Here's how the part is built. I have some questions about the finished solid (model axes, mm). Face numbers are marked on the shaded views. A direction names the side the tool comes from. Coordinates: 2 decimals unless noted, no trailing zeros. Order: outer loops, then holes, each group sorted by start corner. A loop starts at its lowest first (then second) coordinate and runs counter-clockwise, first axis right, second up. Notation, with made-up numbers: (14.25, 45.5) - (52.25, 45.5) arc R6 ccw to (52.25, 53.5) - close; hole circle Ø9 at (-11.5, 13). An arc over 180 degrees is marked (long way). Answer as CSV lines item,"result". Start each with the question number.
Item 1: I'm going to push flat-ended pins straight in: pin 1 (10 mm diameter, centred on y = -380.5, z = 182.5, fed in from -X); pin 2 (12 mm diameter, centred on x = 169.5, y = -310, fed in from -Z); pin 3 (8 mm diameter, centred on x = 40, y = -347, fed in from +Z). Where does each tip first touch, or does it pass through?
Item 2: I need wall thicknesses on line 1 (Z direction, x = 0, y = -113); line 2 (X direction, y = -492.5, z = 32); line 3 (Z direction, x = 149.5, y = -647.7). Which ranges of each line are inside material? Lowest first, please.
Item 3: Imagine slicing it at C-C on x = 0. List the corners of the cut face in (y, z) for me.
Item 4: On a 3-axis mill with a long thin cutter (end or side, diameter ignored), from which of +Z, -Z, +X, -X, +Y, -Y can I reach the whole of each face in a straight line? I mean the marked faces 1, 2 and 3. Say none if no direction works.
Item 5: Imagine slicing it at D-D on z = 0. List the corners of the cut face in (x, y) for me, and give its area (3 significant figures).
Item 6: We'd pull the mould along Z, two halves only. Please class the marked faces 4, 5, 6 and 7: pulls with the +Z half, pulls with the -Z half, needs draft (parallel to the pull), parting line crosses it, or undercut.
Item 7: Imagine slicing it at A-A on y = -647.7. List the corners of the cut face in (x, z) for me.
Item 8: Imagine slicing it at B-B on y = -482. List the corners of the cut face in (x, z) for me.
from build123d import *

# Parameters (mm, degrees)
F0_R     = 254
F0_R_2   = 127
F1_DEPTH = 254
F2_R     = 254
F3_DEPTH = 127
F4_W     = 112.5292529635
F4_H     = 228.6
F5_DEPTH = 381
F6_R     = 38.1
F7_DEPTH = 480.8302529635


with BuildPart() as f1:
    # F0 (on Front) → F1 (new body)
    with BuildSketch(Plane.XZ):
        Circle(F0_R)
        Circle(F0_R_2, mode=Mode.SUBTRACT)
    extrude(amount=F1_DEPTH)

    # F2 (on face) → F3 (join)
    with BuildSketch(Plane.XZ.offset(254)):
        Circle(F2_R)
    extrude(amount=F3_DEPTH)

    # F4 (on face) → F5 (join)
    with BuildSketch(Plane.XZ.offset(381)):
        with Locations((-170.5646264818, 0)):
            Rectangle(F4_W, F4_H)
        with Locations((170.5646264818, 0)):
            Rectangle(F4_W, F4_H)
    extrude(amount=F5_DEPTH)

    # F6 (on face) → F7 (cut, through all)
    with BuildSketch(Plane.YZ.offset(226.8292529635)):
        with Locations((-647.7, 0)):
            Circle(F6_R)
    extrude(amount=-F7_DEPTH, mode=Mode.SUBTRACT)


solid = f1.part
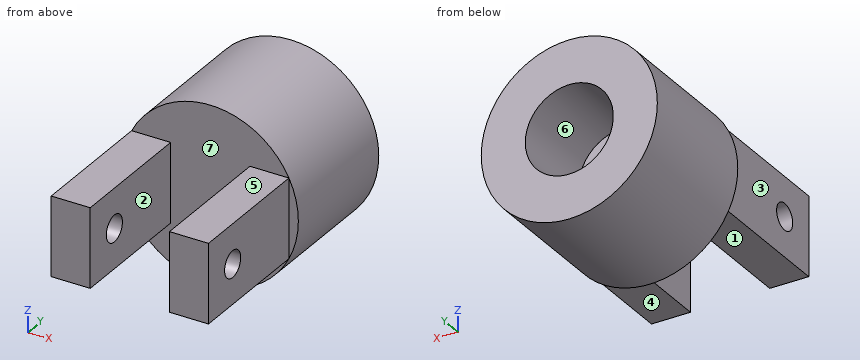
Responses:
1,pin 1,"stops at x = -181.69"
1,pin 2,"stops at z = -194.38"
1,pin 3,"stops at z = 251.44"
2,line 1,"z = -254 to -127, 127 to 254"
2,line 2,"x = -226.83 to -114.3, 114.3 to 226.83"
2,line 3,"z = -114.3 to -38.1, 38.1 to 114.3"
3,outline,"(-381, -254) - (0, -254) - (0, -127) - (-254, -127) - (-254, 127) - (0, 127) - (0, 254) - (-381, 254) - close"
4,face 1,"-Z, +X, -X, -Y"
4,face 2,"+Z, -Z, -Y"
4,face 3,"+Z, -Z, -X, -Y"
5,outline,"(-254, -381) - (-226.83, -381) - (-226.83, -609.6) - (-114.3, -609.6) - (-114.3, -381) - (114.3, -381) - (114.3, -609.6) - (226.83, -609.6) - (226.83, -381) - (254, -381) - (254, 0) - (127, 0) - (127, -254) - (-127, -254) - (-127, 0) - (-254, 0) - close; (-226.83, -762) - (-114.3, -762) - (-114.3, -685.8) - (-226.83, -685.8) - close; (114.3, -762) - (226.83, -762) - (226.83, -685.8) - (114.3, -685.8) - close"
5,area,"198,000 mm^2"
6,face 4,"pulls with the -Z half"
6,face 5,"pulls with the +Z half"
6,face 6,"undercut"
6,face 7,"needs draft"
7,outline,"(-226.83, -114.3) - (-114.3, -114.3) - (-114.3, -38.1) - (-226.83, -38.1) - close; (-226.83, 38.1) - (-114.3, 38.1) - (-114.3, 114.3) - (-226.83, 114.3) - close; (114.3, -114.3) - (226.83, -114.3) - (226.83, -38.1) - (114.3, -38.1) - close; (114.3, 38.1) - (226.83, 38.1) - (226.83, 114.3) - (114.3, 114.3) - close"
8,outline,"(-226.83, -114.3) - (-114.3, -114.3) - (-114.3, 114.3) - (-226.83, 114.3) - close; (114.3, -114.3) - (226.83, -114.3) - (226.83, 114.3) - (114.3, 114.3) - close"
